Check sheet for the drawn part. Datum: minimum x, y, z corner. Units: mm. Round coordinates to 2 decimals unless told otherwise and drop trailing zeros. Write each loop counter-clockwise with the first axis right and the second up, starting at its lowest first coordinate (ties: lowest second). Pieces come first, ordered by that corner, then holes.
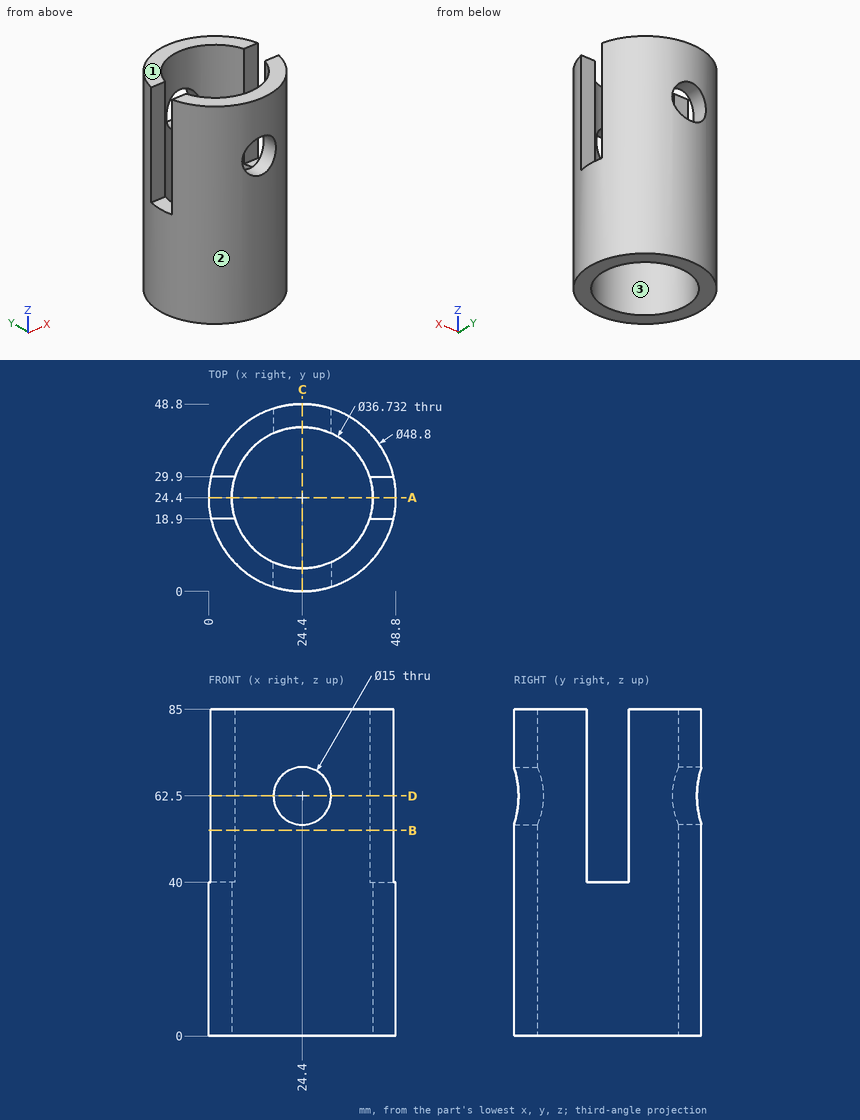
Q1. Sectioned sample at C-C (x = 24.4). Enter the section's corners in (y, z).
Recorded:
outline: (0, 0) - (6.03, 0) - (6.03, 55) - (0, 55) - close; (0, 70) - (6.03, 70) - (6.03, 85) - (0, 85) - close; (42.77, 0) - (48.8, 0) - (48.8, 55) - (42.77, 55) - close; (42.77, 70) - (48.8, 70) - (48.8, 85) - (42.77, 85) - close
Q2. Sectioned sample at B-B (z = 53.5). Enter the section's corners in (x, y).
Recorded:
outline: (0.63, 18.9) arc R24.4 ccw to (48.17, 18.9) - (41.92, 18.9) arc R18.37 cw to (6.88, 18.9) - close; (0.63, 29.9) - (6.88, 29.9) arc R18.37 cw to (41.92, 29.9) - (48.17, 29.9) arc R24.4 ccw to start
Q3. Sectioned sample at D-D (z = 62.5). Enter the section's corners in (x, y) (1 decimal), plus the area to 3 significant figures.
Recorded:
outline: (0.6, 18.9) arc R24.4 ccw to (16.9, 1.2) - (16.9, 7.6) arc R18.4 cw to (6.9, 18.9) - close; (0.6, 29.9) - (6.9, 29.9) arc R18.4 cw to (16.9, 41.2) - (16.9, 47.6) arc R24.4 ccw to start; (31.9, 1.2) arc R24.4 ccw to (48.2, 18.9) - (41.9, 18.9) arc R18.4 cw to (31.9, 7.6) - close; (31.9, 41.2) arc R18.4 cw to (41.9, 29.9) - (48.2, 29.9) arc R24.4 ccw to (31.9, 47.6) - close
area: 491 mm2
Q4. Material ranges on line 1 along Z through (x, y) = (24.4, 46); line 2 along X through (y, z) = (24.5, 26.5) (1 decimal); line 3 along Y through (x, z) = (46, 53.5), recorded low to high.
Recorded:
line 1: z = 0 to 55, 70 to 85
line 2: x = 0 to 6, 42.8 to 48.8
line 3: y = 13.05 to 18.9, 29.9 to 35.75
Q5. Sectioned sample at A-A (y = 24.4). Enter the section's corners in (x, z), plus the area to 3 significant figures.
Recorded:
outline: (0, 0) - (6.03, 0) - (6.03, 40) - (0, 40) - close; (42.77, 0) - (48.8, 0) - (48.8, 40) - (42.77, 40) - close
area: 483 mm2
Q6. Release check for a two-part mould opening along Y. For the marked faces 1, 2 and 3 record: released by +Y, released by -Y, zero draft, split by the parting line, or undercut.
Recorded:
face 1: zero draft
face 2: split by the parting line
face 3: undercut
Q7. Depth check by flat-ended pin: P1, Ø5.5, axis at x = 3.5, y = 22.5, coming from the +Z side; P2, Ø1, axis at y = 25.5, z = 14.5, coming from the -X side; P3, Ø5, axis at x = 3, z = 53, coming from the -Y side. Enter the tip coordinate at first touch or a pass-through.
Recorded:
P1: stops at z = 40
P2: stops at x = 0.01
P3: stops at y = 8.97
